from build123d import *

# Parameters (mm, degrees)
F0_W     = 146.409407258
F0_H     = 121.9511963427
F1_DEPTH = 127
F4_D     = 25.4
F2_W     = 146.409407258
F2_H     = 121.9511963427
F2_R     = 20.4523292797
F6_DEPTH = 127


with BuildPart() as f1:
    # F0 (on Front) → F1 (new body)
    with BuildSketch(Plane.XZ):
        with Locations((-1.3189986348, -14.5600493997)):
            Rectangle(F0_W, F0_H)
    extrude(amount=F1_DEPTH)

    # F4 (through all)
    with Locations(Plane(origin=(0, 0, 0), x_dir=(-1, 0, 0), z_dir=(0, 1, 0))):
        with Locations((-28.0630998313, -46.4930534363)):
            Hole(F4_D / 2)


with BuildPart() as f6:
    # F2 (on face) → F6 (new body)
    with BuildSketch(Plane(origin=(0, 0, 0), x_dir=(-1, 0, 0), z_dir=(0, 1, 0))):
        with Locations((1.3189986348, -14.5600493997)):
            Rectangle(F2_W, F2_H)
        with Locations((-28.8153458387, -45.7823053002)):
            Circle(F2_R, mode=Mode.SUBTRACT)
    extrude(amount=F6_DEPTH)


solid = f6.part
Part model, mm, in its own coordinate system. Round coordinates to 2 decimals unless told otherwise and drop trailing zeros. Loops run counter-clockwise (first coordinate to the right, second up) from the corner with the lowest first, then second, coordinate; pieces in that order, holes last. Notation, with made-up numbers: (28, 29) - (33, 29) arc R24 cw to (33, 48) - close; hole circle Ø5 at (44, 31.5). An arc over 180 degrees is marked (long way). Answer as a JSON object with one key per item and string values.
Item 1: Pin check, flat tip, straight feed: pin 1 (2 mm diameter, centred on x = -40, z = 25, fed in from -Y). Stop position of the tip, or through.
Output:
{"pin 1": "y = 0"}
Item 2: Band-saw the part on B-B on y = 89. List the corners of the cut face in (x, z).
Output:
{"outline": "(-74.52, -75.54) - (71.89, -75.54) - (71.89, 46.42) - (-74.52, 46.42) - close; hole circle Ø40.9 at (28.82, -45.78)"}
Item 3: Pull direction Z, two halves, no side cores. Call faces 1 (the face through (0, 63, 46.416)), 2 (the face through (9.307, 62.611, -39.639)), 3 (the face through (0, 63, -75.536)), 4 (the face through (-74.524, 63, -15)): pulls with the +Z half, pulls with the -Z half, needs draft (parallel to the pull), parting line crosses it, or undercut.
Output:
{"face 1": "pulls with the +Z half", "face 2": "undercut", "face 3": "pulls with the -Z half", "face 4": "needs draft"}
Item 4: Band-saw the part on A-A on z = -51. List the corners of the cut face in (x, y), plus the area to 3 significant figures.
Output:
{"outline": "(-74.52, 0) - (9.04, 0) - (9.04, 127) - (-74.52, 127) - close; (48.59, 0) - (71.89, 0) - (71.89, 127) - (48.59, 127) - close", "area": "13,600 mm2"}
Item 5: Wall check: L1, parallel to X at y = 31.5, z = -43; L2, parallel to X at y = 16.5, z = -60; L3, parallel to Z at x = 18, y = 73. Give the ranges that are in metal, low to high.
Output:
{"L1": "-74.52 to 8.55, 49.08 to 71.89", "L2": "-74.52 to 14.11, 43.52 to 71.89", "L3": "-75.54 to -63.14, -28.42 to 46.42"}
